Can you work these out from the model? Positions are in its coordinate system, mm. A direction names the side the tool comes from. Give positions to 0.01 mm unless a question says otherwise; leave off trailing zeros. Write each loop counter-clockwise with the first axis right and the second up, starting at its lowest first coordinate (ties: lowest second). Pieces come first, ordered by that corner, then holes.
```python
from build123d import *

# Parameters (mm, degrees)
BOSS_EXTRUDE1_DEPTH     = 25.4
CUT_EXTRUDE3_REACH      = 349.398
FILLET1_R               = 1.27
CUT_EXTRUDE4_REACH      = 333.236
SKETCH4_R               = 4.7625
FILLET2_R               = 12.7
CUT_EXTRUDE5_DEPTH      = 332.236354444
CUT_EXTRUDE5_DEPTH_BACK = 332.236354444
SKETCH17_R              = 4.7625
SKETCH18_W              = 68.58
SKETCH18_H              = 17.78
SKETCH18_W_2            = 17.78
SKETCH18_H_2            = 43.18
CUT_EXTRUDE6_DEPTH      = 19.05
FILLET3_R               = 6.35


with BuildPart() as part:
    # Sketch1 → Boss-Extrude1 (new body)
    with BuildSketch(Plane(origin=(0, 0, 0), x_dir=(1, 0, 0), z_dir=(0, 1, 0))):
        with BuildLine():
            Line((44.45, -6.35), (184.15, -6.35))
            ThreePointArc((184.15, -6.35), (197.620384182, -0.770384182), (203.2, 12.7))
            Line((203.2, 12.7), (203.2, 44.45))
            Line((203.2, 44.45), (228.6, 44.45))
            Line((228.6, 44.45), (228.6, -260.35))
            Line((228.6, -260.35), (203.2, -260.35))
            Line((203.2, -260.35), (203.2, -50.8))
            ThreePointArc((203.2, -50.8), (197.620384182, -37.329615818), (184.15, -31.75))
            Line((184.15, -31.75), (19.05, -31.75))
            ThreePointArc((19.05, -31.75), (5.579615818, -26.170384182), (0, -12.7))
            Line((0, -12.7), (0, 44.45))
            Line((0, 44.45), (25.4, 44.45))
            Line((25.4, 44.45), (25.4, 12.7))
            ThreePointArc((25.4, 12.7), (30.979615818, -0.770384182), (44.45, -6.35))
        make_face()
    extrude(amount=BOSS_EXTRUDE1_DEPTH)

    # Sketch3 → Cut-Extrude3 (cut, up to next)
    with BuildSketch(Plane(origin=(0, 25.4, 0), x_dir=(1, 0, 0), z_dir=(0, 1, 0)), mode=Mode.PRIVATE) as cut_extrude3_sk1:
        Polygon((215.9, -260.35), (228.6, -260.35), (228.6, -152.4), (227.33, -152.4), (204.47, -260.35), align=None)
    cut_extrude3_tool1 = extrude(cut_extrude3_sk1.sketch, amount=-CUT_EXTRUDE3_REACH, mode=Mode.PRIVATE) & part.part
    add(cut_extrude3_tool1.solids().sort_by_distance((220.5355, 25.4, 222.5675))[0], mode=Mode.SUBTRACT)

    # Fillet1
    fillet1_edges = [part.edges().sort_by_distance(p)[0] for p in [
        (0, 12.7, -44.45),
        (25.4, 12.7, -44.45),
        (203.2, 12.7, -44.45),
        (228.6, 12.7, -44.45),
        (228.6, 0, 53.975),
        (203.2, 0, 155.575),
        (197.620384182, 0, 37.329615818),
        (5.579615818, 0, 26.170384182),
        (101.6, 0, 31.75),
        (197.620384182, 0, 0.770384182),
        (203.2, 0, -28.575),
        (114.3, 0, 6.35),
        (30.979615818, 0, 0.770384182),
        (25.4, 0, -28.575),
        (0, 0, -15.875),
        (25.4, 25.4, -28.575),
        (30.979615818, 25.4, 0.770384182),
        (114.3, 25.4, 6.35),
        (197.620384182, 25.4, 0.770384182),
        (203.2, 25.4, -28.575),
        (228.6, 25.4, 53.975),
        (203.2, 25.4, 155.575),
        (197.620384182, 25.4, 37.329615818),
        (101.6, 25.4, 31.75),
        (5.579615818, 25.4, 26.170384182),
        (0, 25.4, -15.875),
    ]]
    fillet(fillet1_edges, radius=FILLET1_R)

    # Cut-Extrude4: up to this plane
    cut_extrude4_end = Plane(origin=(248.460888859, -0.001, 52.615247053), z_dir=(-0.9783048645494203, 0, -0.20717044190458336))
    # Sketch4 → Cut-Extrude4 (cut, up to the surface)
    with BuildSketch(Plane.ZY.offset(-203.2), mode=Mode.PRIVATE) as cut_extrude4_sk1:
        with BuildLine():
            ThreePointArc((182.5625, 12.7), (177.8, 17.4625), (173.0375, 12.7))
            Line((173.0375, 12.7), (182.5625, 12.7))
        make_face()
    cut_extrude4_tool1 = split(extrude(cut_extrude4_sk1.sketch, amount=-CUT_EXTRUDE4_REACH, mode=Mode.PRIVATE), bisect_by=cut_extrude4_end, keep=Keep.BOTH, mode=Mode.PRIVATE)
    add(cut_extrude4_tool1.solids().sort_by_distance((203.2, 14.721268, 177.8))[0], mode=Mode.SUBTRACT)
    # Sketch4 → Cut-Extrude4 (cut, up to the surface)
    with BuildSketch(Plane.ZY.offset(-203.2), mode=Mode.PRIVATE) as cut_extrude4_sk2:
        with BuildLine():
            Line((182.5625, 12.7), (173.0375, 12.7))
            ThreePointArc((173.0375, 12.7), (177.8, 7.9375), (182.5625, 12.7))
        make_face()
    cut_extrude4_tool2 = split(extrude(cut_extrude4_sk2.sketch, amount=-CUT_EXTRUDE4_REACH, mode=Mode.PRIVATE), bisect_by=cut_extrude4_end, keep=Keep.BOTH, mode=Mode.PRIVATE)
    add(cut_extrude4_tool2.solids().sort_by_distance((203.2, 10.678732, 177.8))[0], mode=Mode.SUBTRACT)
    # Sketch4 → Cut-Extrude4 (cut, up to the surface)
    with BuildSketch(Plane.ZY.offset(-203.2), mode=Mode.PRIVATE) as cut_extrude4_sk3:
        with BuildLine():
            ThreePointArc((182.5625, 12.7), (177.8, 17.4625), (173.0375, 12.7))
            Line((173.0375, 12.7), (182.5625, 12.7))
        make_face()
    cut_extrude4_tool3 = split(extrude(cut_extrude4_sk3.sketch, amount=-CUT_EXTRUDE4_REACH, mode=Mode.PRIVATE), bisect_by=cut_extrude4_end, keep=Keep.BOTH, mode=Mode.PRIVATE)
    add(cut_extrude4_tool3.solids().sort_by_distance((203.2, 14.721268, 177.8))[0], mode=Mode.SUBTRACT)
    # Sketch4 → Cut-Extrude4 (cut, up to the surface)
    with BuildSketch(Plane.ZY.offset(-203.2), mode=Mode.PRIVATE) as cut_extrude4_sk4:
        with BuildLine():
            Line((182.5625, 12.7), (173.0375, 12.7))
            ThreePointArc((173.0375, 12.7), (177.8, 7.9375), (182.5625, 12.7))
        make_face()
    cut_extrude4_tool4 = split(extrude(cut_extrude4_sk4.sketch, amount=-CUT_EXTRUDE4_REACH, mode=Mode.PRIVATE), bisect_by=cut_extrude4_end, keep=Keep.BOTH, mode=Mode.PRIVATE)
    add(cut_extrude4_tool4.solids().sort_by_distance((203.2, 10.678732, 177.8))[0], mode=Mode.SUBTRACT)
    # Sketch4 → Cut-Extrude4 (cut, up to the surface)
    with BuildSketch(Plane.ZY.offset(-203.2), mode=Mode.PRIVATE) as cut_extrude4_sk5:
        with Locations((234.95, 12.7)):
            Circle(SKETCH4_R)
    cut_extrude4_tool5 = split(extrude(cut_extrude4_sk5.sketch, amount=-CUT_EXTRUDE4_REACH, mode=Mode.PRIVATE), bisect_by=cut_extrude4_end, keep=Keep.BOTH, mode=Mode.PRIVATE)
    add(cut_extrude4_tool5.solids().sort_by_distance((203.2, 12.7, 234.95))[0], mode=Mode.SUBTRACT)

    # Fillet2
    # the kernel refuses this fillet: 12.7 mm, written as the material it takes off along each edge
    with BuildSketch(Plane(origin=(0, 12.7, -31.75), x_dir=(0, 1, 0), z_dir=(0, 0, 1))) as fillet2_piece_1:
        with BuildLine():
            CenterArc((11.43, -1.27), 1.27, 0, 90)
            Line((12.7, -1.27), (12.7, 0))
            Line((12.7, 0), (11.43, 0))
        make_face()
    revolve(axis=Axis((0, 12.7, -31.75), (-1, 0, 0)), revolution_arc=90, mode=Mode.SUBTRACT)
    with BuildSketch(Plane(origin=(25.4, 12.7, -31.75), x_dir=(0, 0, -1), z_dir=(0, -1, 0))) as fillet2_piece_2:
        with BuildLine():
            CenterArc((11.43, -1.27), 1.27, 0, 90)
            Line((12.7, -1.27), (12.7, 0))
            Line((12.7, 0), (11.43, 0))
        make_face()
    revolve(axis=Axis((25.4, 12.7, -31.75), (1, 0, 0)), revolution_arc=90, mode=Mode.SUBTRACT)
    with BuildSketch(Plane(origin=(203.2, 12.7, -31.75), x_dir=(0, 0, -1), z_dir=(0, 1, 0))) as fillet2_piece_3:
        with BuildLine():
            CenterArc((11.43, -1.27), 1.27, 0, 90)
            Line((12.7, -1.27), (12.7, 0))
            Line((12.7, 0), (11.43, 0))
        make_face()
    revolve(axis=Axis((203.2, 12.7, -31.75), (-1, 0, 0)), revolution_arc=90, mode=Mode.SUBTRACT)
    with BuildSketch(Plane(origin=(228.6, 12.7, -31.75), x_dir=(0, -1, 0), z_dir=(0, 0, 1))) as fillet2_piece_4:
        with BuildLine():
            CenterArc((11.43, -1.27), 1.27, 0, 90)
            Line((12.7, -1.27), (12.7, 0))
            Line((12.7, 0), (11.43, 0))
        make_face()
    revolve(axis=Axis((228.6, 12.7, -31.75), (1, 0, 0)), revolution_arc=90, mode=Mode.SUBTRACT)
    with BuildSketch(Plane(origin=(203.2, 12.7, -31.75), x_dir=(0, 1, 0), z_dir=(0, 0, 1))) as fillet2_piece_5:
        with BuildLine():
            CenterArc((11.43, -1.27), 1.27, 0, 90)
            Line((12.7, -1.27), (12.7, 0))
            Line((12.7, 0), (11.43, 0))
        make_face()
    revolve(axis=Axis((203.2, 12.7, -31.75), (-1, 0, 0)), revolution_arc=90, mode=Mode.SUBTRACT)
    with BuildSketch(Plane(origin=(228.6, 12.7, -31.75), x_dir=(0, 0, -1), z_dir=(0, -1, 0))) as fillet2_piece_6:
        with BuildLine():
            CenterArc((11.43, -1.27), 1.27, 0, 90)
            Line((12.7, -1.27), (12.7, 0))
            Line((12.7, 0), (11.43, 0))
        make_face()
    revolve(axis=Axis((228.6, 12.7, -31.75), (1, 0, 0)), revolution_arc=90, mode=Mode.SUBTRACT)
    with BuildSketch(Plane(origin=(0, 12.7, -31.75), x_dir=(0, 0, -1), z_dir=(0, 1, 0))) as fillet2_piece_7:
        with BuildLine():
            CenterArc((11.43, -1.27), 1.27, 0, 90)
            Line((12.7, -1.27), (12.7, 0))
            Line((12.7, 0), (11.43, 0))
        make_face()
    revolve(axis=Axis((0, 12.7, -31.75), (-1, 0, 0)), revolution_arc=90, mode=Mode.SUBTRACT)
    with BuildSketch(Plane(origin=(25.4, 12.7, -31.75), x_dir=(0, -1, 0), z_dir=(0, 0, 1))) as fillet2_piece_8:
        with BuildLine():
            CenterArc((11.43, -1.27), 1.27, 0, 90)
            Line((12.7, -1.27), (12.7, 0))
            Line((12.7, 0), (11.43, 0))
        make_face()
    revolve(axis=Axis((25.4, 12.7, -31.75), (1, 0, 0)), revolution_arc=90, mode=Mode.SUBTRACT)
    with BuildSketch(Plane(origin=(203.2, 25.4, -44.45), x_dir=(0, 0, 1), z_dir=(1, 0, 0)), Plane(origin=(0, 25.4, -44.45), x_dir=(0, 0, 1), z_dir=(1, 0, 0))) as fillet2_piece_9:
        with BuildLine():
            CenterArc((FILLET2_R, FILLET2_R), FILLET2_R, 180, 90)
            Line((0, FILLET2_R), (0, 0))
            Line((0, 0), (FILLET2_R, 0))
        make_face()
    extrude(amount=25.4, mode=Mode.SUBTRACT)
    with BuildSketch(Plane(origin=(203.2, 0, -44.45), x_dir=(0, 0, 1), z_dir=(1, 0, 0)), Plane(origin=(0, 0, -44.45), x_dir=(0, 0, 1), z_dir=(1, 0, 0))) as fillet2_piece_10:
        with BuildLine():
            CenterArc((FILLET2_R, -FILLET2_R), FILLET2_R, 90, 90)
            Line((0, -FILLET2_R), (0, 0))
            Line((0, 0), (FILLET2_R, 0))
        make_face()
    extrude(amount=25.4, mode=Mode.SUBTRACT)

    # Sketch17 → Cut-Extrude5 (cut, two sides: drawn at the far end of the back side and taken through both)
    with BuildSketch(Plane.ZY.offset(-203.2).offset(-CUT_EXTRUDE5_DEPTH_BACK)):
        with Locations((-27.94, 12.7)):
            Circle(SKETCH17_R)
    extrude(amount=CUT_EXTRUDE5_DEPTH + CUT_EXTRUDE5_DEPTH_BACK, mode=Mode.SUBTRACT)

    # Sketch18 → Cut-Extrude6 (cut)
    with BuildSketch(Plane(origin=(0, 25.4, 0), x_dir=(1, 0, 0), z_dir=(0, 1, 0))):
        with Locations((78.74, -19.05)):
            Rectangle(SKETCH18_W, SKETCH18_H)
        with Locations((149.86, -19.05)):
            Rectangle(SKETCH18_W, SKETCH18_H)
        with Locations((215.9, -72.39)):
            Rectangle(SKETCH18_W_2, SKETCH18_H_2)
        with Locations((215.9, -118.11)):
            Rectangle(SKETCH18_W_2, SKETCH18_H_2)
    extrude(amount=-CUT_EXTRUDE6_DEPTH, mode=Mode.SUBTRACT)

    # Fillet3
    fillet3_edges = [part.edges().sort_by_distance(p)[0] for p in [
        (224.79, 15.875, 96.52),
        (224.79, 15.875, 139.7),
        (207.01, 15.875, 139.7),
        (207.01, 15.875, 96.52),
        (224.79, 15.875, 50.8),
        (224.79, 15.875, 93.98),
        (207.01, 15.875, 93.98),
        (207.01, 15.875, 50.8),
        (115.57, 15.875, 10.16),
        (184.15, 15.875, 10.16),
        (184.15, 15.875, 27.94),
        (115.57, 15.875, 27.94),
        (113.03, 15.875, 10.16),
        (113.03, 15.875, 27.94),
        (44.45, 15.875, 27.94),
        (44.45, 15.875, 10.16),
    ]]
    fillet(fillet3_edges, radius=FILLET3_R)


solid = part.part
```
1) For pin 1 Ø4 at (x, y) = (138.5, 11.5) entering from -Z; pin 2 Ø2 at (y, z) = (5, 41) entering from -X; pin 3 Ø2 at (x, y) = (186.5, 9.5) entering from -Z, each with a flat end and sliding along its axis, tell me the tip position at first contact or that it passes through.
Values follow:
pin 1: stops at z = 6.35
pin 2: stops at x = 199.84
pin 3: stops at z = 6.05
2) Suppose I cut it at B-B on z = 234.95. Write out the boundary of the cut face in (x, y).
Values follow:
outline: (203.2, 1.27) arc R1.27 ccw to (204.47, 0) - (209.85, 0) - (209.85, 7.94) - (203.2, 7.94) - close; (203.2, 17.46) - (209.85, 17.46) - (209.85, 25.4) - (204.47, 25.4) arc R1.27 ccw to (203.2, 24.13) - close
3) Suppose I cut it at A-A on z = -27.94. Write out the boundary of the cut face in (x, y).
Values follow:
outline: (0, 1.27) arc R1.27 ccw to (1.27, 0) - (24.13, 0) arc R1.27 ccw to (25.4, 1.27) - (25.4, 7.94) - (0, 7.94) - close; (0, 17.46) - (25.4, 17.46) - (25.4, 24.13) arc R1.27 ccw to (24.13, 25.4) - (1.27, 25.4) arc R1.27 ccw to (0, 24.13) - close; (203.2, 1.27) arc R1.27 ccw to (204.47, 0) - (227.33, 0) arc R1.27 ccw to (228.6, 1.27) - (228.6, 7.94) - (203.2, 7.94) - close; (203.2, 17.46) - (228.6, 17.46) - (228.6, 24.13) arc R1.27 ccw to (227.33, 25.4) - (204.47, 25.4) arc R1.27 ccw to (203.2, 24.13) - close
4) Suppose I cut it at C-C on x = 128.5. Write out the boundary of the cut face in (y, z), plus the area to 3 significant figures.
Values follow:
outline: (0, 7.62) arc R1.27 ccw to (1.27, 6.35) - (24.13, 6.35) arc R1.27 ccw to (25.4, 7.62) - (25.4, 10.16) - (6.35, 10.16) - (6.35, 27.94) - (25.4, 27.94) - (25.4, 30.48) arc R1.27 ccw to (24.13, 31.75) - (1.27, 31.75) arc R1.27 ccw to (0, 30.48) - close
area: 305 mm2
5) Suppose I cut it at D-D on z = 77. Write out the boundary of the cut face in (x, y).
Values follow:
outline: (203.2, 1.27) arc R1.27 ccw to (204.47, 0) - (227.33, 0) arc R1.27 ccw to (228.6, 1.27) - (228.6, 24.13) arc R1.27 ccw to (227.33, 25.4) - (224.79, 25.4) - (224.79, 6.35) - (207.01, 6.35) - (207.01, 25.4) - (204.47, 25.4) arc R1.27 ccw to (203.2, 24.13) - close
6) If we mould it in two halves opening along Y, with no side actions, what happens to faces 1 (the face through (12.9, 12.9, -32.7)), 2 (the face through (149, 6.35, 19)), 3 (the face through (113, 13, 6.35)), 4 (the face through (206.16, 12.909, 230.192))? For each: +Y half, -Y half, draft (parallel to the pull), parting line (faces both ways), or undercut.
Values follow:
face 1: undercut
face 2: +Y half
face 3: draft
face 4: undercut
7) For faces 5 (the face through (30.83, 12.54, 0.62)), 6 (the face through (208.82, 15.74, 92.07)), 7 (the face through (228.6, 13, 53)), which set-ups out of +Z, -Z, +X, -X, +Y, -Y let a thin tool reach every point of the face, with its end or its side?
Values follow:
face 5: -Z, +Y, -Y
face 6: +Y
face 7: +Z, -Z, +X, +Y, -Y
8) Please list where these lines run through material, in increasing order: L1, parallel to Z at x = 150, y = 7.5; L2, parallel to Z at x = 209.25, y = 12.7; L3, parallel to Y at x = 215, z = -27.94.
Values follow:
L1: z = 6.35 to 10.16, 27.94 to 31.75
L2: z = -44.45 to -32.7, -23.18 to 52.31, 92.47 to 98.03, 138.19 to 173.04, 182.56 to 230.19
L3: y = 0 to 7.94, 17.46 to 25.4
